Can you work these out from the model? Positions are in its coordinate system, mm. Coordinates: 2 decimals unless noted, no trailing zeros. Loops run counter-clockwise (first coordinate to the right, second up) from the corner with the lowest first, then second, coordinate; pieces in that order, holes last. Notation, with made-up numbers: M 2.25,83 L 24.25,83 A19 cw 24.25,91 Z; hole C -8.5,63 d10. An arc over 180 degrees is marked long. Return JSON: item names as keys, results as strings. Group by question number.
```python
from build123d import *

# Parameters (mm, degrees)
SKETCH5_R           = 35
SKETCH5_R_2         = 1.75
BOSS_EXTRUDE2_DEPTH = 6
FILLET1_R           = 30
CIRPATTERN3_DEPTH   = 6


# Read off the part's stored shape, not the designer's step: CirPattern3
with BuildPart() as part:
    # Sketch5 → Boss-Extrude2 (new body)
    with BuildSketch(Plane.XY):
        Polygon((-40, 60), (40, 60), (71.961524227, 4.641016151), (31.961524227, -64.641016151), (-31.961524227, -64.641016151), (-71.961524227, 4.641016151), align=None)
        Circle(SKETCH5_R, mode=Mode.SUBTRACT)
        with Locations((-25, 52)):
            Circle(SKETCH5_R_2, mode=Mode.SUBTRACT)
        with Locations((25, 52)):
            Circle(SKETCH5_R_2, mode=Mode.SUBTRACT)
        with Locations((57.533320997, -4.349364905)):
            Circle(SKETCH5_R_2, mode=Mode.SUBTRACT)
        with Locations((32.533320997, -47.650635095)):
            Circle(SKETCH5_R_2, mode=Mode.SUBTRACT)
        with Locations((-32.533320997, -47.650635095)):
            Circle(SKETCH5_R_2, mode=Mode.SUBTRACT)
        with Locations((-57.533320997, -4.349364905)):
            Circle(SKETCH5_R_2, mode=Mode.SUBTRACT)
    extrude(amount=BOSS_EXTRUDE2_DEPTH)

    # Fillet1
    fillet1_edges = [part.edges().sort_by_distance(p)[0] for p in [
        (-40, 60, 3),
        (40, 60, 3),
    ]]
    fillet(fillet1_edges, radius=FILLET1_R)

    # CirPattern3 outline → CirPattern3 (cut)
    with BuildSketch(Plane.XY):
        with BuildLine():
            Line((-71.961524227, 4.641016151), (-63.301270189, -10.358983849))
            ThreePointArc((-63.301270189, -10.358983849), (-67.320508076, 4.641016151), (-63.301270189, 19.641016151))
            Line((-63.301270189, 19.641016151), (-71.961524227, 4.641016151))
        make_face()
        with BuildLine():
            Line((-31.961524227, -64.641016151), (-14.641016151, -64.641016151))
            ThreePointArc((-14.641016151, -64.641016151), (-29.641016151, -60.621778265), (-40.621778265, -49.641016151))
            Line((-40.621778265, -49.641016151), (-31.961524227, -64.641016151))
        make_face()
        with BuildLine():
            Line((31.961524227, -64.641016151), (40.621778265, -49.641016151))
            ThreePointArc((40.621778265, -49.641016151), (29.641016151, -60.621778265), (14.641016151, -64.641016151))
            Line((14.641016151, -64.641016151), (31.961524227, -64.641016151))
        make_face()
        with BuildLine():
            ThreePointArc((63.301270189, 19.641016151), (67.320508076, 4.641016151), (63.301270189, -10.358983849))
            Line((63.301270189, -10.358983849), (71.961524227, 4.641016151))
            Line((71.961524227, 4.641016151), (63.301270189, 19.641016151))
        make_face()
    extrude(amount=CIRPATTERN3_DEPTH, mode=Mode.SUBTRACT)


solid = part.part
```
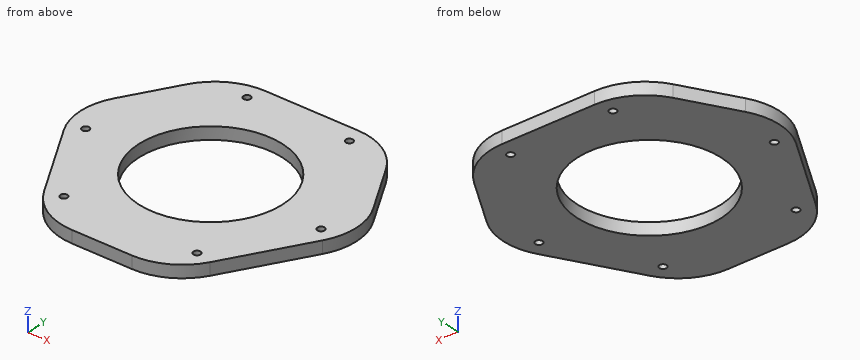
1) Suppose I cut it at A-A, the plane x = -25. List the corners of the cut face in (y, z) for me.
2) Suppose I cut it at D-D, the plane x = 0. List the corners of the cut face in (y, z) for me, then the cut area to 3 significant figures.
3) Suppose I cut it at B-B, the plane y = -31. List the corners of the cut face in (x, z) for me.
4) If I drill on line 1 (Y direction, x = 0, z = 2.8); line 2 (X direction, y = 18, z = 2.8); line 3 (Y direction, x = -25, z = 3.7), over which ranges is the centre line in solid material (lowest first)? Write a range as from..to.
5) Suppose I cut it at C-C, the plane z = 2.2. List the corners of the cut face in (x, y) for me, then the cut area to 3 significant figures.
6) For pin 1 (4.5 mm diameter, centred on x = -25, y = 52, fed in from -Z); pin 2 (3 mm diameter, centred on x = 32.53, y = -47.65, fed in from +Z); pin 3 (1.5 mm diameter, centred on y = -49, z = 3.5, fed in from +X); pin 4 (1.5 mm diameter, centred on x = -30, z = 3, fed in from +Y), each with a flat end and sliding along its axis, tell me the tip position at first contact or that it passes through.
Returned:
{
 "1": {"outline": "M -62.8,0 L -24.49,0 L -24.49,6 L -62.8,6 Z; M 24.49,0 L 50.25,0 L 50.25,6 L 24.49,6 Z; M 53.75,0 L 59.91,0 L 59.91,6 L 53.75,6 Z"},
 "2": {"outline": "M -64.64,0 L -35,0 L -35,6 L -64.64,6 Z; M 35,0 L 60,0 L 60,6 L 35,6 Z", "area": "328 mm²"},
 "3": {"outline": "M -51.38,0 L -16.25,0 L -16.25,6 L -51.38,6 Z; M 16.25,0 L 51.38,0 L 51.38,6 L 16.25,6 Z"},
 "4": {"line 1": "y = -64.64..-35, 35..60", "line 2": "x = -64.18..-30.02, 30.02..64.18", "line 3": "y = -62.8..-24.49, 24.49..50.25, 53.75..59.91"},
 "5": {"outline": "M -63.3,-10.36 L -40.62,-49.64 A30 ccw -14.64,-64.64 L 14.64,-64.64 A30 ccw 40.62,-49.64 L 63.3,-10.36 A30 ccw 63.3,19.64 L 48.66,45 A30 ccw 22.68,60 L -22.68,60 A30 ccw -48.66,45 L -63.3,19.64 A30 ccw Z; hole C -57.53,-4.35 d3.5; hole C 0,0 d70; hole C -32.53,-47.65 d3.5; hole C -25,52 d3.5; hole C 25,52 d3.5; hole C 32.53,-47.65 d3.5; hole C 57.53,-4.35 d3.5", "area": "9,200 mm²"},
 "6": {"pin 1": "stops at z = 0", "pin 2": "passes through", "pin 3": "stops at x = 41.42", "pin 4": "stops at y = 59.27"}
}
